Input: part model. Units: mm. Frame: model coordinates. Coordinates: 2 decimals unless noted, no trailing zeros. Order: outer loops, then holes, each group sorted by start corner. A loop starts at its lowest first (then second) coordinate and runs counter-clockwise, first axis right, second up. Notation, with made-up numbers: M 25.25,20.25 L 82.25,20.25 A13 ccw 82.25,24.25 Z; hole C 79.5,43 d8. An arc over 180 degrees is marked long. Answer in a Markdown table with one row per item.
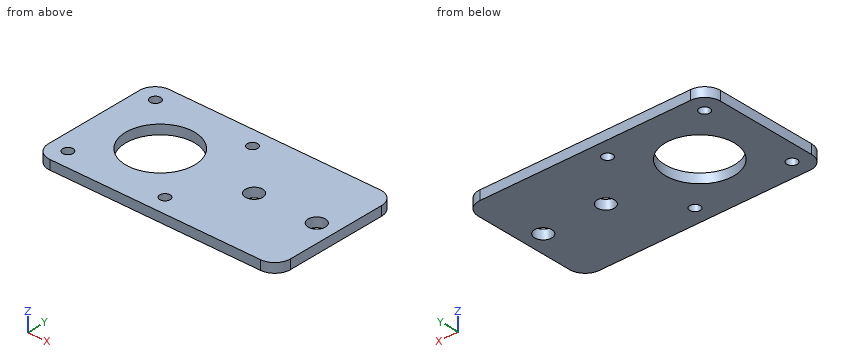
from build123d import *

# Parameters (mm, degrees)
F1_DEPTH = 3
F3_D     = 3.3
F5_D     = 5.5
F6_R     = 5


with BuildPart() as f1:
    # F0 (on Top) → F1 (new body)
    with BuildSketch(Plane.XY):
        Polygon((0, 21.15), (0, 0), (77.3, 0), (77.3, 42.3), (0, 42.3), align=None)
        with BuildLine():
            ThreePointArc((32.15, 21.15), (21.15, 10.15), (10.15, 21.15))
            ThreePointArc((10.15, 21.15), (21.15, 32.15), (32.15, 21.15))
        make_face(mode=Mode.SUBTRACT)
    extrude(amount=F1_DEPTH)

    # F3 (through all)
    with Locations(Plane.XY.offset(3)):
        with Locations((5.65, 36.65), (36.65, 36.65), (36.65, 5.65), (5.65, 5.65)):
            Hole(F3_D / 2)

    # F5 (through all)
    with Locations(Plane.XY.offset(3)):
        with Locations((51.15, 21.15), (71.15, 21.15)):
            Hole(F5_D / 2)

    # F6
    f6_edges = [f1.edges().sort_by_distance(p)[0] for p in [
        (77.3, 0, 1.5),
        (0, 0, 1.5),
        (77.3, 42.3, 1.5),
        (0, 42.3, 1.5),
    ]]
    fillet(f6_edges, radius=F6_R)


solid = f1.part
1) Cut plane B-B, the plane z = 1. Output: boundary loops of the cut face in (x, y), and give its area (3 significant figures).
Resolved:
| item | result |
|---|---|
| outline | M 0,5 A5 ccw 5,0 L 72.3,0 A5 ccw 77.3,5 L 77.3,37.3 A5 ccw 72.3,42.3 L 5,42.3 A5 ccw 0,37.3 Z; hole C 5.65,5.65 d3.3; hole C 5.65,36.65 d3.3; hole C 21.15,21.15 d22; hole C 36.65,5.65 d3.3; hole C 36.65,36.65 d3.3; hole C 51.15,21.15 d5.5; hole C 71.15,21.15 d5.5 |
| area | 2,790 mm2 |
2) Material intervals for probe 1 along Y at (x, z) = (36.65, 2.15); probe 2 along X at (y, z) = (5.5, 0.9); probe 3 along X at (y, z) = (23, 1.2), sorted ascending.
Resolved:
| item | result |
|---|---|
| probe 1 | y = 0 to 4, 7.3 to 35, 38.3 to 42.3 |
| probe 2 | x = 0 to 4.01, 7.29 to 35.01, 38.29 to 77.3 |
| probe 3 | x = 0 to 10.31, 31.99 to 49.12, 53.18 to 69.12, 73.18 to 77.3 |
3) Cut plane A-A, the plane x = 21.15. Output: boundary loops of the cut face in (y, z).
Resolved:
| item | result |
|---|---|
| outline | M 0,0 L 10.15,0 L 10.15,3 L 0,3 Z; M 32.15,0 L 42.3,0 L 42.3,3 L 32.15,3 Z |
4) Cut plane C-C, the plane y = 21.15. Output: boundary loops of the cut face in (x, z), and give its area (3 significant figures).
Resolved:
| item | result |
|---|---|
| outline | M 0,0 L 10.15,0 L 10.15,3 L 0,3 Z; M 32.15,0 L 48.4,0 L 48.4,3 L 32.15,3 Z; M 53.9,0 L 68.4,0 L 68.4,3 L 53.9,3 Z; M 73.9,0 L 77.3,0 L 77.3,3 L 73.9,3 Z |
| area | 133 mm2 |
5) Cut plane D-D, the plane y = 31. Output: boundary loops of the cut face in (x, z).
Resolved:
| item | result |
|---|---|
| outline | M 0,0 L 16.25,0 L 16.25,3 L 0,3 Z; M 26.05,0 L 77.3,0 L 77.3,3 L 26.05,3 Z |
